from build123d import *

# Parameters (mm, degrees)
PAD_DEPTH       = 28
FILLET_R        = 2
SKETCH003_R     = 2.1
POCKET001_DEPTH = 10


with BuildPart() as part:
    # Sketch → Pad (new body, symmetric)
    with BuildSketch(Plane.YZ):
        Polygon((-2, 4.125), (3.4, 4.125), (3.4, 6.95), (12.65, 6.95), (12.65, -6.95), (3.4, -6.95), (3.4, -4.125), (-2, -4.125), align=None)
    extrude(amount=PAD_DEPTH, both=True)

    # Fillet
    fillet_edges = [part.edges().sort_by_distance(p)[0] for p in [
        (-28, 8.025, 6.95),
        (0, 3.4, 6.95),
        (0, 12.65, 6.95),
        (28, 8.025, 6.95),
        (28, 12.65, 0),
        (0, 12.65, -6.95),
        (-28, 12.65, 0),
        (-28, 8.025, -6.95),
        (28, 8.025, -6.95),
        (0, 3.4, -6.95),
        (28, 3.4, -5.5375),
        (28, 3.4, 5.5375),
        (-28, 3.4, -5.5375),
        (-28, 0.7, -4.125),
        (28, 0.7, -4.125),
        (28, 0.7, 4.125),
        (-28, 0.7, 4.125),
        (-28, 3.4, 5.5375),
    ]]
    fillet(fillet_edges, radius=FILLET_R)

    # Sketch003 (on Face2 of Fillet) → Pocket001 (cut)
    with BuildSketch(Plane(origin=(0, -2, 0), x_dir=(0, 0, -1), z_dir=(0, -1, 0))):
        with Locations((0, 20)):
            Circle(SKETCH003_R)
        with Locations((0, -20)):
            Circle(SKETCH003_R)
    extrude(amount=-POCKET001_DEPTH, mode=Mode.SUBTRACT)


solid = part.part
Design review of the part built by this model. Coordinates are the model's own, in mm. A direction names the side the tool comes from. Coordinates: 2 decimals unless noted, no trailing zeros. Loops run counter-clockwise (first coordinate to the right, second up) from the corner with the lowest first, then second, coordinate; pieces in that order, holes last. Notation, with made-up numbers: M -11.75,66.5 L 7.25,66.5 A16 cw 7.25,97.5 Z; hole C 21.5,40.25 d7. An arc over 180 degrees is marked long. Use one line per item in the form item = value.
(1) Consider section D-D (x = 20). Write out the cut boundary in (y, z) (3 decimals).
Return value:
outline = M -2,-4.125 L 3.4,-4.125 L 3.4,-4.95 A2 ccw 5.4,-6.95 L 10.65,-6.95 A2 ccw 12.65,-4.95 L 12.65,4.95 A2 ccw 10.65,6.95 L 5.4,6.95 A2 ccw 3.4,4.95 L 3.4,4.125 L -2,4.125 L -2,2.1 L 8,2.1 L 8,-2.1 L -2,-2.1 Z
(2) Consider section C-C (z = 0). Write out the cut boundary in (x, y).
Return value:
outline = M -28,-2 L -22.1,-2 L -22.1,8 L -17.9,8 L -17.9,-2 L 17.9,-2 L 17.9,8 L 22.1,8 L 22.1,-2 L 28,-2 L 28,10.65 A2 ccw 26,12.65 L -26,12.65 A2 ccw -28,10.65 Z
(3) Clearance check with flat-ended pins moving along their axes: P1, Ø4, axis at x = -20, y = 1, coming from the +Z side (3 decimals); P2, Ø1.5, axis at x = 3.5, y = 1.5, coming from the -Z side (3 decimals); P3, Ø6, axis at x = -7, y = 2, coming from the -Z side. State where each tip first meets the part, or that it passes through.
Return value:
P1 = 4.125
P2 = -4.125
P3 = -6.91
(4) Consider section B-B (x = 8). Write out the cut boundary in (y, z) (3 decimals), and give its area (3 significant figures).
Return value:
outline = M -2,-4.125 L 3.4,-4.125 L 3.4,-4.95 A2 ccw 5.4,-6.95 L 10.65,-6.95 A2 ccw 12.65,-4.95 L 12.65,4.95 A2 ccw 10.65,6.95 L 5.4,6.95 A2 ccw 3.4,4.95 L 3.4,4.125 L -2,4.125 Z
area = 170 mm2
(5) Draft analysis for pull direction Z (two halves, no side actions). For faces 5 (the face through (-27.399, 0.93, 3.555)), 6 (the face through (-28, 6, 0)), 7 (the face through (-18.23, 2.93, -1.13)), state which applies: pulls with the +Z half, pulls with the -Z half, needs draft (parallel to the pull), parting line crosses it, or undercut.
Return value:
face_5 = pulls with the +Z half
face_6 = needs draft
face_7 = undercut
(6) For line 1 along X through (y, z) = (4, 0); line 2 along X through (y, z) = (2.5, -0.5); line 3 along Z through (x, y) = (-3, 3.25) (3 decimals), list the stretches that pass through material, from the lowest coordinate up. Write a range as from..to.
Return value:
line_1 = -28..-22.1, -17.9..17.9, 22.1..28
line_2 = -28..-22.04, -17.96..17.96, 22.04..28
line_3 = -4.125..4.125
(7) For faces 1 (the face through (27.65, 4.27, 4.19)), 2 (the face through (0, 1, 4.125)), 3 (the face through (21.77, 2.93, -1.13)), 4 (the face through (27.65, 4.27, -4.15)), list the 3-axis set-ups (+Z, -Z, +X, -X, +Y, -Y) from which the entire face can be reached by the end or side of a thin tool; tool diameter is ignored.
Return value:
face_1 = +Z, +X, -Y
face_2 = +Z, +X, -X, -Y
face_3 = -Y
face_4 = -Z, +X, -Y
(8) Consider section A-A (y = 0.25). Write out the cut boundary in (x, z) (3 decimals).
Return value:
outline = M -28,-2.125 A2 ccw -26,-4.125 L 26,-4.125 A2 ccw 28,-2.125 L 28,2.125 A2 ccw 26,4.125 L -26,4.125 A2 ccw -28,2.125 Z; hole C -20,0 d4.2; hole C 20,0 d4.2
